Check sheet for the modelled part. Datum: model origin and axes. Units: mm. Face numbers are marked on the shaded views. Coordinates: 2 decimals unless noted, no trailing zeros. Write each loop counter-clockwise with the first axis right and the second up, starting at its lowest first coordinate (ties: lowest second). Pieces come first, ordered by that corner, then holes. Notation, with made-up numbers: M -11.75,20.5 L 4.25,20.5 A19 ccw 4.25,26.5 Z; hole C 6.25,43.25 d6. An arc over 180 degrees is marked long. Answer as CSV lines item,"result". Start each with the question number.
1) Section check D-D (z = 12.75). State how many separate pieces and enclosed holes the cut face has, and give its area (3 significant figures).
2) Draft check along X on the marked faces 1 and 2. Enter one of: +X half, -X half, draft (parallel to the pull), parting line (faces both ways), or undercut.
3) Section check C-C (x = -165.5). Record the cut outline in (y, z).
4) Go/stop test with flat-tipped pins: pin 1 Ø3 at (y, z) = (-67.5, 18.5) entering from -X; pin 2 Ø12 at (y, z) = (-141.5, 8) entering from -X; pin 3 Ø3 at (x, z) = (-101, 10) entering from -Y. Record where each tip stops, or that it passes through.
5) Material ranges on L1, parallel to Y at x = -130, z = 21; L2, parallel to Y at x = -131, z = 13.5; L3, parallel to Y at x = 9, z = 10, recorded low to high. Write a range as [from, to].
6) Section check B-B (x = -34). Record the cut outline in (y, z).
7) Section check A-A (y = 21). Record the cut outline in (x, z) (3 decimals).
from build123d import *

# Parameters (mm, degrees)
F0_R     = 54.4924805174
F0_R_2   = 43.1604920117
F0_R_3   = 47.1840335611
F0_R_4   = 46.467
F1_DEPTH = 25
F3_DEPTH = 25
F4_R     = 5


with BuildPart() as f1:
    # F0 (on Top) → F1 (new body)
    with BuildSketch(Plane.XY):
        with BuildLine():
            ThreePointArc((-171.1951607712, -99.3221294101), (-127.2895477252, -199.5524067975), (-60.162123745, -113.1364342468))
            ThreePointArc((-60.162123745, -113.1364342468), (27.5666162737, -88.5949500771), (-48.7532108312, -38.8566322407))
            ThreePointArc((-48.7532108312, -38.8566322407), (-95.9689877261, 38.3611262057), (-155.4748304215, -29.836868577))
            ThreePointArc((-155.4748304215, -29.836868577), (-259.0763673914, -42.9189917909), (-171.1951607712, -99.3221294101))
        make_face()
        with Locations((-119.4296146298, -136.3778748382)):
            Circle(F0_R, mode=Mode.SUBTRACT)
        with Locations((-21.8538418412, -81.0042768717)):
            Circle(F0_R_2, mode=Mode.SUBTRACT)
        with Locations((-204.9019783735, -55.1753938198)):
            Circle(F0_R_3, mode=Mode.SUBTRACT)
        with BuildLine():
            ThreePointArc((-159.087277872, -86.5775758158), (-150.3684240565, -65.719362224), (-150.6837491193, -43.1144057719))
            ThreePointArc((-150.6837491193, -43.1144057719), (-114.4142534505, -72.0060826257), (-68.7840436754, -63.7544607623))
            ThreePointArc((-68.7840436754, -63.7544607623), (-71.8518551472, -80.5585578366), (-69.0841155831, -97.4146773015))
            ThreePointArc((-69.0841155831, -97.4146773015), (-111.819217091, -73.1727968314), (-159.087277872, -86.5775758158))
        make_face(mode=Mode.SUBTRACT)
        with Locations((-100.6964207948, -17.5737444198)):
            Circle(F0_R_4, mode=Mode.SUBTRACT)
    extrude(amount=F1_DEPTH)

    # F2 (on face) → F3 (join)
    with BuildSketch(Plane.XY.offset(25)):
        with BuildLine():
            ThreePointArc((-127.7027924667, 87.8290782041), (-71.8303532525, 121.9260893446), (-92.3607341122, 59.7743468572))
            ThreePointArc((-92.3607341122, 59.7743468572), (-104.6730727654, 52.5942964384), (-105.4238538636, 38.3611262057))
            ThreePointArc((-105.4238538636, 38.3611262057), (-98.4279417265, 38.5146891297), (-91.4672809773, 37.7966570014))
            Line((-91.4672809773, 37.7966570014), (-95.1554035699, 41.0152669471))
            ThreePointArc((-95.1554035699, 41.0152669471), (-96.5776784553, 46.4608516232), (-92.0321108024, 49.7797479798))
            ThreePointArc((-92.0321108024, 49.7797479798), (-65.6130297513, 129.7583871225), (-137.5112819177, 85.881378358))
            ThreePointArc((-137.5112819177, 85.881378358), (-131.6331872692, 81.9509835556), (-127.7027924667, 87.8290782041))
        make_face()
    extrude(amount=-F3_DEPTH)

    # F4
    f4_edges = [f1.edges().sort_by_distance(p)[0] for p in [
        (-105.423854, 38.361126, 12.5),
        (-91.467281, 37.796657, 12.5),
    ]]
    fillet(f4_edges, radius=F4_R)


solid = f1.part
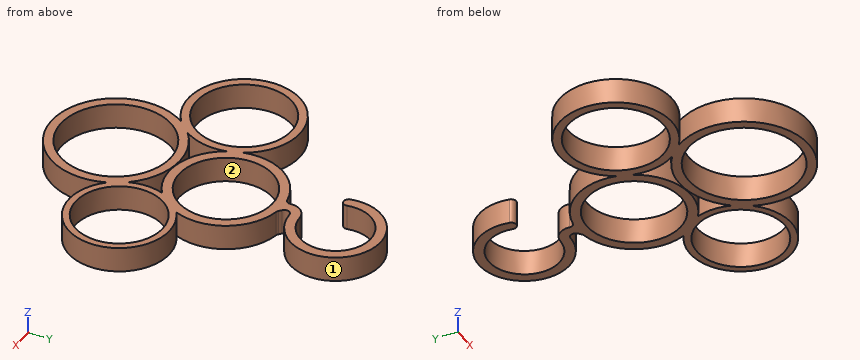
Results found:
1,separate pieces,"1"
1,enclosed holes,"5"
1,area,"13,300 mm2"
2,face 1,"parting line"
2,face 2,"undercut"
3,outline,"M -180.31,0 L -165.48,0 L -165.48,25 L -180.31,25 Z; M -107.28,0 L -81.13,0 L -81.13,25 L -107.28,25 Z; M -29.22,0 L -16.03,0 L -16.03,25 L -29.22,25 Z"
4,pin 1,"stops at x = -259.38"
4,pin 2,"stops at x = -183.09"
4,pin 3,"stops at y = -197.75"
5,L1,"y = [-199.16, -189.84], [-82.92, -73.6], [-65.45, -53.64], [18.49, 30.3], [82.59, 120.72]"
5,L2,"y = [-198.98, -189.63], [-83.13, -73.78], [-64.83, -52.8], [17.65, 29.68], [82.12, 119.26]"
5,L3,"y = [-120.35, -111.18], [-50.82, -41.66]"
6,outline,"M -129.51,0 L -122.42,0 L -122.42,25 L -129.51,25 Z; M -39.59,0 L -32.5,0 L -32.5,25 L -39.59,25 Z"
7,outline,"M -141.478,0 L -126.605,0 L -126.605,25 L -141.478,25 Z; M -74.788,0 L -59.915,0 L -59.915,25 L -74.788,25 Z"
